Design review of the part built by this model. Coordinates are the model's own, in mm. A direction names the side the tool comes from. Round coordinates to 2 decimals unless told otherwise and drop trailing zeros. Order: outer loops, then holes, each group sorted by start corner. A loop starts at its lowest first (then second) coordinate and runs counter-clockwise, first axis right, second up. Notation, with made-up numbers: (40, 54.5) - (97, 54.5) arc R18 ccw to (97, 81.5) - close; hole circle Ø10 at (59, -23.5). An arc over 180 degrees is marked (long way). Use CSV: the item, a comma, the result in double quotes.
from build123d import *

# Parameters (mm, degrees)
BOSS_EXTRUDE1_DEPTH = 20
CHAMFER1_SIZE       = 1
SKETCH2_W           = 3
SKETCH2_H           = 5.519803574
CUT_EXTRUDE1_DEPTH  = 26


with BuildPart() as part:
    # Sketch1 → Boss-Extrude1 (new body)
    with BuildSketch(Plane(origin=(0, 0, 0), x_dir=(1, 0, 0), z_dir=(0, 1, 0))):
        Polygon((0.084907706, 6.13), (-5.266281872, 3.13853223), (-5.351189578, -2.99146777), (-0.084907706, -6.13), (5.266281872, -3.13853223), (5.351189578, 2.99146777), align=None)
        Polygon((0.041549541, 2.999712259), (-2.57705225, 1.535839087), (-2.618601791, -1.463873171), (-0.041549541, -2.999712259), (2.57705225, -1.535839087), (2.618601791, 1.463873171), align=None, mode=Mode.SUBTRACT)
    extrude(amount=BOSS_EXTRUDE1_DEPTH)

    # Chamfer1
    chamfer1_edges = [part.edges().sort_by_distance(p)[0] for p in [
        (1.330075666, 0, -2.231792715),
        (-1.267751354, 0, -2.267775673),
        (-2.59782702, 0, -0.035982958),
        (-1.330075666, 0, 2.231792715),
        (1.267751354, 0, 2.267775673),
        (2.59782702, 0, 0.035982958),
        (1.330075666, 20, -2.231792715),
        (-1.267751354, 20, -2.267775673),
        (-2.59782702, 20, -0.035982958),
        (-1.330075666, 20, 2.231792715),
        (1.267751354, 20, 2.267775673),
        (2.59782702, 20, 0.035982958),
    ]]
    chamfer(chamfer1_edges, length=CHAMFER1_SIZE)

    # Sketch2 → Cut-Extrude1 (cut)
    with BuildSketch(Plane(origin=(0, 20, 0), x_dir=(1, 0, 0), z_dir=(0, 1, 0))):
        with Locations((-0.084907706, -4.416905982)):
            Rectangle(SKETCH2_W, SKETCH2_H)
    extrude(amount=-CUT_EXTRUDE1_DEPTH, mode=Mode.SUBTRACT)


solid = part.part
1) We need section D-D (z = -3.5). Give the boundary of the cut face in (x, y).
Data:
outline,"(-4.62, 0) - (-1.11, 0) - (0.05, 0.57) - (1.16, 0) - (4.5, 0) - (4.5, 20) - (1.16, 20) - (0.05, 19.43) - (-1.11, 20) - (-4.62, 20) - close"
2) We need section C-C (y = 1.5). Give the boundary of the cut face in (x, z).
Data:
outline,"(-5.35, 2.99) - (-5.27, -3.14) - (0.08, -6.13) - (5.35, -2.99) - (5.27, 3.14) - (1.42, 5.29) - (1.42, 2.19) - (2.58, 1.54) - (2.62, -1.46) - (0.04, -3) - (-2.58, -1.54) - (-2.62, 1.46) - (-1.58, 2.08) - (-1.58, 5.24) - close"
3) For faces 1 (the face through (1.35, 9.87, -2.22)), 2 (the face through (-2.5, 0, -3)), 3 (the face through (1.615, 19.507, -2.652)), 4 (the face through (-2.424, 0.382, 2.299)), list the 3-axis set-ups (+Z, -Z, +X, -X, +Y, -Y) from which the entire face can be reached by the end or side of a thin tool; tool diameter is ignored.
Data:
face 1,"+Y, -Y"
face 2,"+Z, -Z, +X, -X, -Y"
face 3,"+Y"
face 4,"-Y"
4) We need section B-B (z = 1.75). Give the boundary of the cut face in (x, y).
Data:
outline,"(-5.33, 0) - (-3.62, 0) - (-3.13, 0.49) - (-2.14, 1) - (-2.14, 19) - (-3.13, 19.51) - (-3.62, 20) - (-5.33, 20) - close; (2.19, 1) - (2.94, 0.64) - (3.57, 0) - (5.29, 0) - (5.29, 20) - (3.57, 20) - (2.94, 19.36) - (2.19, 19) - close"
5) Insertion check: pin 1 Ø4 at (x, y) = (-2, 13) entering from -Z; pin 2 Ø0.9 at (y, z) = (6.5, 4.5) entering from +X; pin 3 Ø4 at (x, y) = (4, 16) entering from +Z. Each pin has a flat end and moves straight along its axis. Give the tip position at first contact, or say it passes through.
Data:
pin 1,"stops at z = -6.08"
pin 2,"stops at x = 3.64"
pin 3,"stops at z = 4.96"
6) To check wall thickness, follow L1, parallel to X at y = 10.25, z = 2.75; L2, parallel to X at y = 11.25, z = -1.25; L3, parallel to Z at x = -2.5, y = 18.5. State the ranges of each line that lie inside material, in increasing order. Write a range as from..to.
Data:
L1,"x = -5.35..-1.58, 1.42..5.27"
L2,"x = -5.29..-2.58, 2.62..5.33"
L3,"z = -4.68..-1.58, 1.53..4.69"
7) We need section A-A (x = -2.25). Give the boundary of the cut face in (y, z).
Data:
outline,"(0, -4.82) - (20, -4.82) - (20, -2.86) - (19, -1.72) - (1, -1.72) - (0, -2.86) - close; (0, 2.85) - (1, 1.68) - (19, 1.68) - (20, 2.85) - (20, 4.84) - (0, 4.84) - close"
8) The part is to be moulded in two halves that separate along Z. For faces 5 (the face through (1.415, 10, 4)), 6 (the face through (-3.49, 9.86, 4.1)), 7 (the face through (-2.109, 9.874, 1.768)), say which applies: +Z half, -Z half, draft (parallel to the pull), parting line (faces both ways), or undercut.
Data:
face 5,"draft"
face 6,"+Z half"
face 7,"undercut"
